Check sheet for the modelled part. Datum: model origin and axes. Units: mm. A direction names the side the tool comes from. Coordinates: 2 decimals unless noted, no trailing zeros. Loops run counter-clockwise (first coordinate to the right, second up) from the corner with the lowest first, then second, coordinate; pieces in that order, holes last. Notation, with made-up numbers: M -37,41 L -23,41 A22 ccw -23,66 Z; hole C -4,63.25 d8. An arc over 180 degrees is marked long. Return JSON: item names as keys, results as strings.
from build123d import *

# Parameters (mm, degrees)
SKETCH1_W           = 60
SKETCH1_H           = 70
BOSS_EXTRUDE1_DEPTH = 30
SHELL1_T            = 2.5


with BuildPart() as part:
    # Sketch1 → Boss-Extrude1 (new body)
    with BuildSketch(Plane.XY):
        Rectangle(SKETCH1_W, SKETCH1_H)
    extrude(amount=BOSS_EXTRUDE1_DEPTH)

    # Shell1 (no face opened: a closed hollow body)
    add(offset(amount=-SHELL1_T, mode=Mode.PRIVATE), mode=Mode.SUBTRACT)


solid = part.part
1) Section check B-B on z = 9. Record the cut outline in (x, y), then the cut area to 3 significant figures.
Answers:
{"outline": "M -30,-35 L 30,-35 L 30,35 L -30,35 Z; hole M -27.5,-32.5 L 27.5,-32.5 L 27.5,32.5 L -27.5,32.5 Z", "area": "625 mm²"}
2) Draft check along Y on faces 3 (the face through (0, 0, 0)), 4 (the face through (0, 35, 15)), 5 (the face through (-27.5, 0, 15)), 6 (the face through (0, -35, 15)). Enter one of: +Y half, -Y half, draft (parallel to the pull), parting line (faces both ways), or undercut.
Answers:
{"face 3": "draft", "face 4": "+Y half", "face 5": "undercut", "face 6": "-Y half"}
3) Set-up check for faces 1 (the face through (0, 0, 30)), 2 (the face through (0, 0, 27.5)): record each of +Z, -Z, +X, -X, +Y, -Y from which the full face is reachable in a straight line by a thin tool's end or side.
Answers:
{"face 1": "+Z, +X, -X, +Y, -Y", "face 2": "none"}
4) Scan lines: line 1 along Y through (x, z) = (-27, 24.75); line 2 along Z through (x, y) = (12, 5.5); line 3 along X through (y, z) = (25, 2.75). Record each from-to range of solid material in increasing order. Write a range as [from, to].
Answers:
{"line 1": "[-35, -32.5], [32.5, 35]", "line 2": "[0, 2.5], [27.5, 30]", "line 3": "[-30, -27.5], [27.5, 30]"}
5) Section check A-A on x = -8.5. Record the cut outline in (y, z), then the cut area to 3 significant figures.
Answers:
{"outline": "M -35,0 L 35,0 L 35,30 L -35,30 Z; hole M -32.5,2.5 L 32.5,2.5 L 32.5,27.5 L -32.5,27.5 Z", "area": "475 mm²"}
